Input: part model. Units: mm. Frame: model coordinates. Face numbers are marked on the shaded views. A direction names the side the tool comes from. Give positions to 0.01 mm unless a question says otherwise; leave off trailing zeros. Loops run counter-clockwise (first coordinate to the right, second up) from the corner with the lowest first, then second, coordinate; pieces in that order, holes last. Notation, with made-up numbers: (39.5, 0.5) - (76.5, 0.5) arc R13 ccw to (76.5, 24.5) - close; hole circle Ø11 at (12.25, 63). An arc over 180 degrees is marked (long way). Answer as a JSON object with one key per item and string values. Group by question number.
(1) Section query D-D (z = 2.75). Return loops of the section in (x, y), plus the area to 3 significant figures.
(2) Material intervals for L1, parallel to Z at x = 4, y = -5.75; L2, parallel to Y at x = -2.75, z = 6.5; L3, parallel to X at y = -4, z = 5, sorted ascending.
(3) Section query A-A (y = 0). Return loops of the section in (x, z).
(4) Pin query (flat end, axial travel): P1, Ø4, axis at x = -2, z = 12, coming from the +Y side; P2, Ø1.5, axis at y = -6, z = 8.5, coming from the -X side; P3, Ø2, axis at x = -3, z = 12, coming from the -Y side. Return the tip coordinate at first contact, or that it passes through.
(5) Access query for the marked faces 1 and 2. Directions: +Z, -Z, +X, -X, +Y, -Y. A direction counts if a zero-diameter tool reaches every point of the face in a straight line with its end or side. Return the directions, or none.
(6) Section query C-C (z = 8). Return loops of the section in (x, y), plus the area to 3 significant figures.
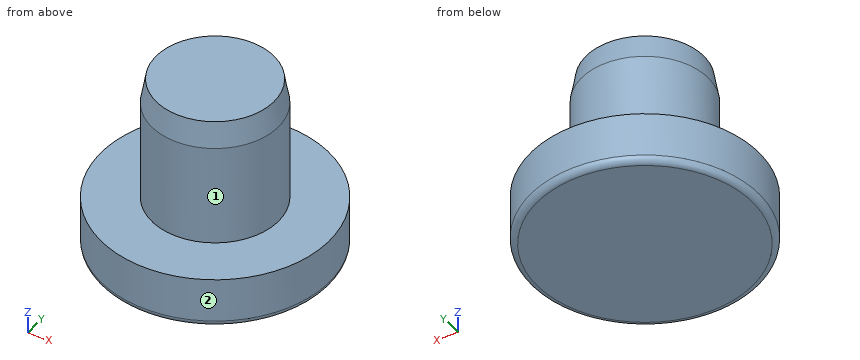
```python
from build123d import *

# Parameters (mm, degrees)
SKETCH_1_R      = 9
EXTRUDE_1_DEPTH = 4
SKETCH_2_R      = 5
EXTRUDE_2_DEPTH = 10
FILLET_1_R      = 0.5
CHAMFER_1_SIZE  = 2
CHAMFER_1_SIZE2 = 0.352653961


with BuildPart() as part:
    # 草图1 → 凸台-拉伸1 (new body)
    with BuildSketch(Plane.XY):
        Circle(SKETCH_1_R)
    extrude(amount=EXTRUDE_1_DEPTH)

    # 草图2 → 凸台-拉伸2 (add)
    with BuildSketch(Plane.XY.offset(4)):
        Circle(SKETCH_2_R)
    extrude(amount=EXTRUDE_2_DEPTH)

    # 圆角1
    fillet_1_edges = [part.edges().sort_by_distance(p)[0] for p in [
        (-9, 0, 0),
    ]]
    fillet(fillet_1_edges, radius=FILLET_1_R)

    # 倒角1
    chamfer_1_edges = [part.edges().sort_by_distance(p)[0] for p in [
        (-5, 0, 14),
    ]]
    chamfer_1_side = [part.faces().sort_by_distance(p)[0] for p in [
        (-5, 0, 9),
    ]]
    chamfer(chamfer_1_edges, length=CHAMFER_1_SIZE, length2=CHAMFER_1_SIZE2, reference=chamfer_1_side[0])


solid = part.part
```
Recorded:
{
 "1": {"outline": "circle Ø18 at (0, 0)", "area": "254 mm^2"},
 "2": {"L1": "z = 0 to 4", "L2": "y = -4.18 to 4.18", "L3": "x = -3 to 3"},
 "3": {"outline": "(-9, 0.5) arc R0.5 ccw to (-8.5, 0) - (8.5, 0) arc R0.5 ccw to (9, 0.5) - (9, 4) - (5, 4) - (5, 12) - (4.65, 14) - (-4.65, 14) - (-5, 12) - (-5, 4) - (-9, 4) - close"},
 "4": {"P1": "stops at y = 5", "P2": "passes through", "P3": "stops at y = -4.58"},
 "5": {"face 1": "+Z", "face 2": "+Z, -Z"},
 "6": {"outline": "circle Ø10 at (0, 0)", "area": "78.5 mm^2"}
}
